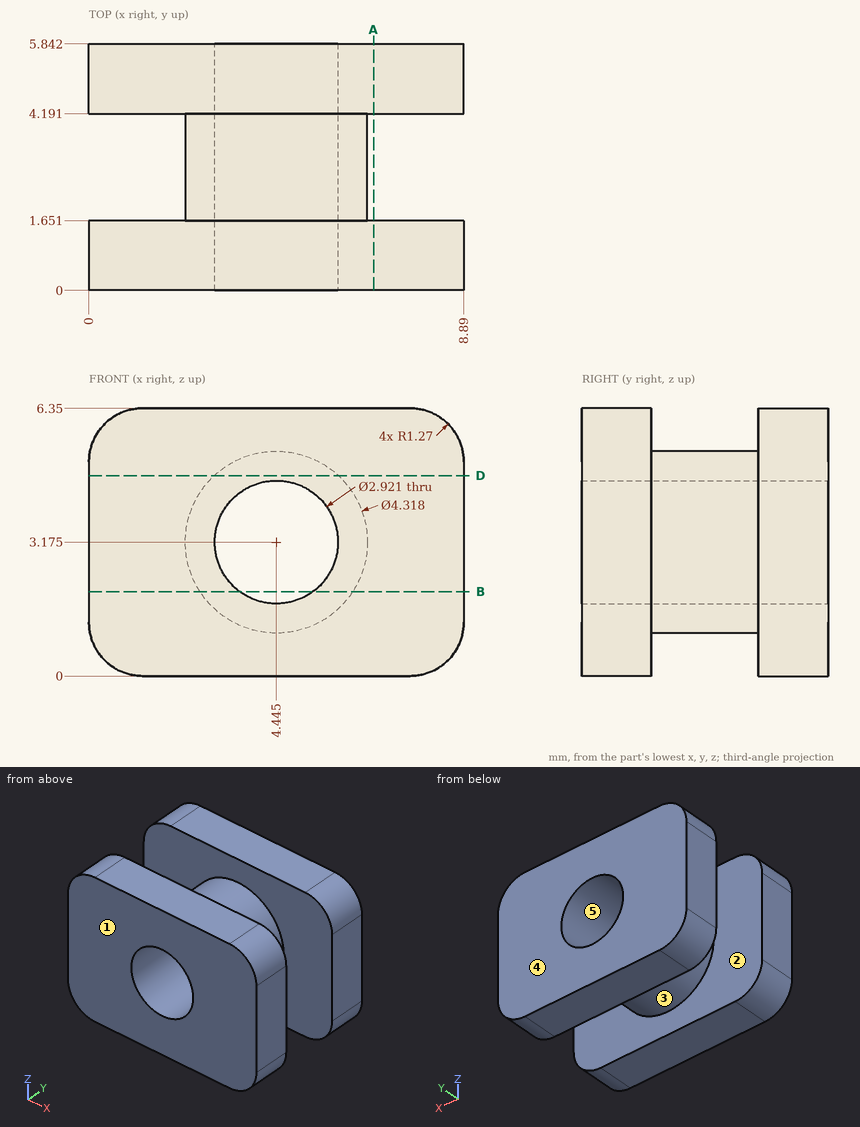
Design review of the part shown in the three views and the two pictorial views. Dimensions are in mm from the part's minimum x, y and z. A direction names the side the tool comes from. Coordinates: 2 decimals unless noted, no trailing zeros. Write each loop counter-clockwise with the first axis right and the second up, starting at its lowest first coordinate (ties: lowest second). Pieces come first, ordered by that corner, then holes.
(1) Tool access review of the marked faces 1 and 2: name each direction out of +Z, -Z, +X, -X, +Y, -Y from which nothing blocks a thin tool from reaching the whole face with its end or side.
(2) The part is to be moulded in two halves that separate along Y. For the marked faces 3, 4 and 5, say which applies: +Y half, -Y half, draft (parallel to the pull), parting line (faces both ways), or undercut.
(3) Add section B-B on z = 2. Give the boundary of the cut face in (x, y), then the cut area to 3 significant figures.
(4) For pin 1 Ø1.8 at (x, z) = (4.445, 3.175) entering from +Y, flat-tipped, find the tip position at first contact; note if it passes through.
(5) Wall thickness on probe 1 along Y at (x, z) = (1.25, 1); probe 2 along Z at (x, y) = (4.5, 0.55); probe 3 along X at (y, z) = (0.9, 2): over which ranges is each line inside the solid? List them lowest first.
(6) Add section D-D on z = 4.75. Give the boundary of the cut face in (x, y).
(7) Add section A-A on x = 6.75. Give the boundary of the cut face in (y, z), then the cut area to 3 significant figures.
Answer sheet:
1. face 1: +Z, -Z, +X, -X, -Y
1. face 2: none
2. face 3: undercut
2. face 4: +Y half
2. face 5: draft
3. outline: (0, 0) - (3.58, 0) - (3.58, 5.84) - (0, 5.84) - (0, 4.19) - (2.63, 4.19) - (2.63, 1.65) - (0, 1.65) - close; (5.31, 0) - (8.89, 0) - (8.89, 1.65) - (6.26, 1.65) - (6.26, 4.19) - (8.89, 4.19) - (8.89, 5.84) - (5.31, 5.84) - close
3. area: 28.4 mm2
4. pin 1: passes through
5. probe 1: y = 0 to 1.65, 4.19 to 5.84
5. probe 2: z = 0 to 1.72, 4.63 to 6.35
5. probe 3: x = 0 to 3.58, 5.31 to 8.89
6. outline: (0, 0) - (8.89, 0) - (8.89, 1.65) - (5.92, 1.65) - (5.92, 4.19) - (8.89, 4.19) - (8.89, 5.84) - (0, 5.84) - (0, 4.19) - (2.97, 4.19) - (2.97, 1.65) - (0, 1.65) - close
7. outline: (0, 0) - (1.65, 0) - (1.65, 6.35) - (0, 6.35) - close; (4.19, 0) - (5.84, 0) - (5.84, 6.35) - (4.19, 6.35) - close
7. area: 21.0 mm2
